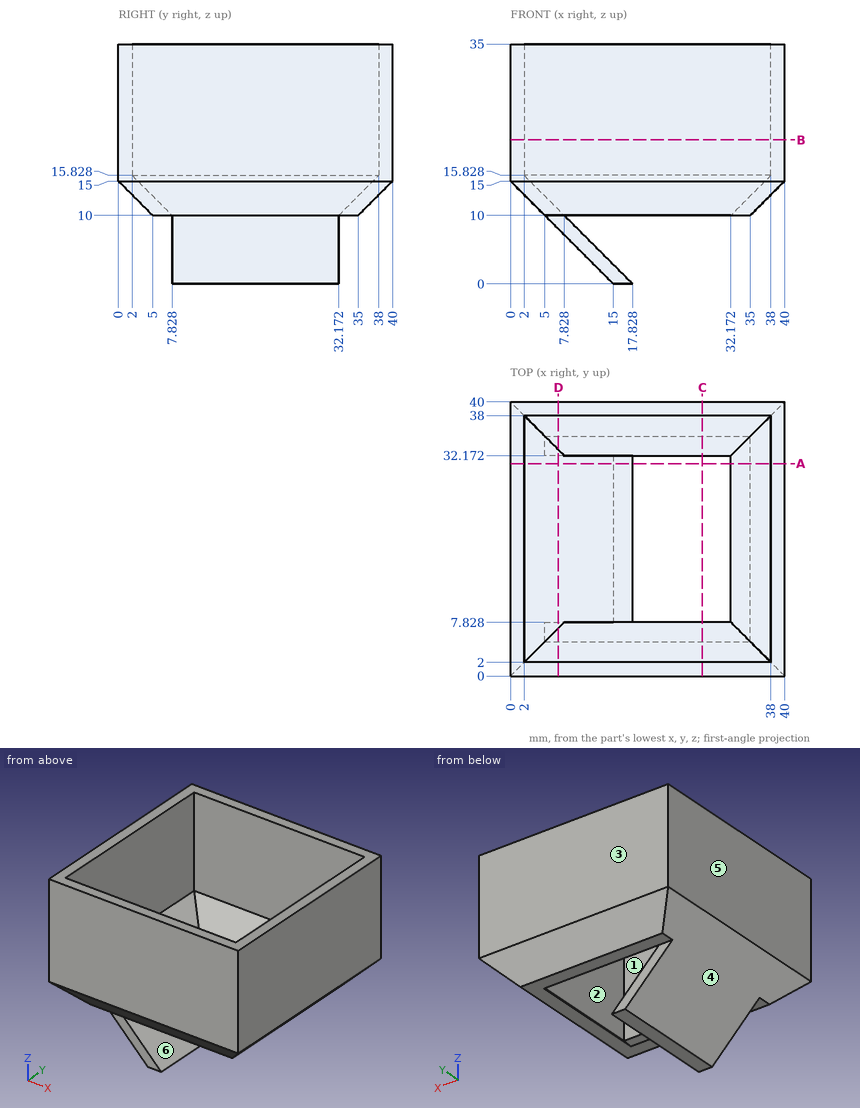
Check sheet for the drawn part. Datum: minimum x, y, z corner. Units: mm. A direction names the side the tool comes from. Round coordinates to 2 decimals unless told otherwise and drop trailing zeros. Loops run counter-clockwise (first coordinate to the right, second up) from the corner with the lowest first, then second, coordinate; pieces in that order, holes last. Notation, with made-up numbers: M 23.25,59.5 L 69.25,59.5 A9 cw 69.25,67.5 Z; hole C -17.5,37.25 d1. An arc over 180 degrees is marked long. One line per question, with ' | ' between items. Start each with the question number.
Item 1: Gauge pin test, flat ends, axial feed: pin 1 Ø8 at (x, z) = (21.5, 9) entering from -Y; pin 2 Ø12 at (x, y) = (6.5, 27.5) entering from -Z; pin 3 Ø8 at (x, z) = (13, 4) entering from -Y. Record the tip position at first contact, or that the pin passes through.
Item 2: Set-up check for the marked faces 5 and 6: record each of +Z, -Z, +X, -X, +Y, -Y from which the full face is reachable in a straight line by a thin tool's end or side.
Item 3: Section check B-B (z = 21). Record the boundary of the cut face in (x, y).
Item 4: Section check C-C (x = 28). Record the boundary of the cut face in (y, z), and give its area (3 significant figures).
Item 5: Section check A-A (y = 31). Record the boundary of the cut face in (x, z).
Item 6: Scan lines: probe 1 along Y at (x, z) = (24, 21); probe 2 along Y at (x, z) = (20, 11). Record each from-to range of solid material in increasing order.
Item 7: Section check D-D (x = 7). Record the boundary of the cut face in (y, z).
Item 8: Release check for a two-part mould opening along Y. For the marked faces 1, 2, 3 and 4 record: released by +Y, released by -Y, zero draft, split by the parting line, or undercut.
Worked out:
1) pin 1: y = 2 | pin 2: z = 2.5 | pin 3: y = 7.83
2) face 5: +Z, -Z, -X, +Y, -Y | face 6: +Z
3) outline: M 0,0 L 40,0 L 40,40 L 0,40 Z; hole M 2,2 L 38,2 L 38,38 L 2,38 Z
4) outline: M 0,15 L 5,10 L 7.83,10 L 2,15.83 L 2,35 L 0,35 Z; M 32.17,10 L 35,10 L 40,15 L 40,35 L 38,35 L 38,15.83 Z | area: 109 mm^2
5) outline: M 0,15 L 15,0 L 17.83,0 L 2,15.83 L 2,35 L 0,35 Z; M 32.17,10 L 35,10 L 40,15 L 40,35 L 38,35 L 38,15.83 Z
6) probe 1: 0 to 2, 38 to 40 | probe 2: 4 to 6.83, 33.17 to 36
7) outline: M 0,15 L 5,10 L 7.83,10 L 7.83,8 L 32.17,8 L 32.17,10 L 35,10 L 40,15 L 40,35 L 38,35 L 38,15.83 L 33,10.83 L 7,10.83 L 2,15.83 L 2,35 L 0,35 Z
8) face 1: undercut | face 2: undercut | face 3: released by +Y | face 4: zero draft
